Design review of the part shown in the three views and the two pictorial views. Dimensions are in mm from the part's minimum x, y and z. Round coordinates to 2 decimals unless told otherwise and drop trailing zeros. Loops run counter-clockwise (first coordinate to the right, second up) from the corner with the lowest first, then second, coordinate; pieces in that order, holes last.
1) Take a section at A-A (z = 0.8). Give the number of separate pieces and of enclosed holes in the cut face, then the cut area to 3 significant figures.
2) Wall thickness on L1, parallel to X at y = 50.5, z = 2.45 (1 decimal); L2, parallel to X at y = 10.5, z = 0.75 (1 decimal); L3, parallel to Y at x = 33.5, z = 1.7: over which ranges is each line inside the solid? List them lowest first.
3) Take a section at C-C (y = 11). State the section outline as (x, z) points (1 decimal), then the cut area to 3 significant figures.
4) Insertion check: pin 1 (3 mm diameter, centred on x = 9.75, y = 92.43, fed in from -Z); pin 2 (3 mm diameter, centred on x = 14, y = 11.5, fed in from -Z). Each pin has a flat end and moves straight along its axis. Give the tip position at first contact, or say it passes through.
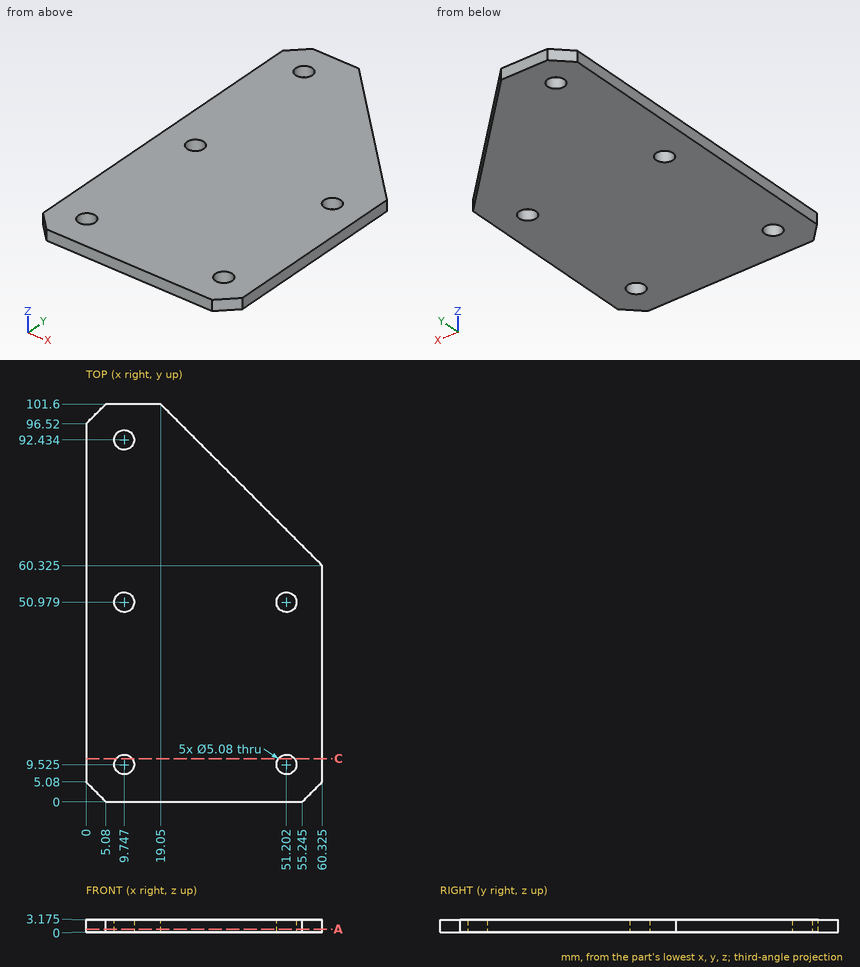
Response:
1. separate pieces: 1
1. enclosed holes: 5
1. area: 5,140 mm2
2. L1: x = 0 to 7.3, 12.2 to 48.7, 53.7 to 60.3
2. L2: x = 0 to 7.4, 12.1 to 48.9, 53.5 to 60.3
2. L3: y = 0 to 87.15
3. outline: (0, 0) - (7.7, 0) - (7.7, 3.2) - (0, 3.2) - close; (11.8, 0) - (49.1, 0) - (49.1, 3.2) - (11.8, 3.2) - close; (53.3, 0) - (60.3, 0) - (60.3, 3.2) - (53.3, 3.2) - close
3. area: 165 mm2
4. pin 1: passes through
4. pin 2: stops at z = 0
